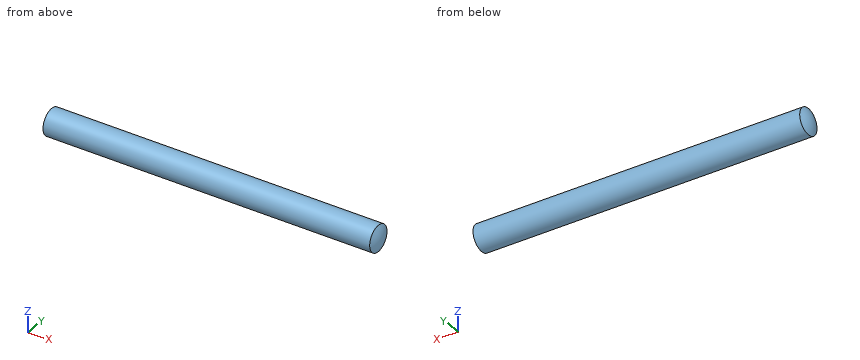
```python
from build123d import *

# Parameters (mm, degrees)
F0_R     = 4
F1_DEPTH = 50


# Not quite as in the source:
# - a pattern or mirror of a feature is missing from the dataset's text; its kind, count and spacing are read off the source's solid


with BuildPart() as f1:
    # F0 (on Right) → F1 (new body, symmetric)
    with BuildSketch(Plane.YZ):
        Circle(F0_R)
    extrude(amount=F1_DEPTH, both=True)

    # F2 (on Front) → F3 (revolve)
    with BuildSketch(Plane.XZ):
        with BuildLine():
            ThreePointArc((51.0717967697, 0), (50.79920338, 2.0705523608), (50, 4))
            Line((50, 4), (50, 0))
            Line((50, 0), (51.0717967697, 0))
        make_face()
    f3 = revolve(axis=Axis((0, 0, 0), (1, 0, 0)))

    # F3_copies: F3 across plane
    add(f3.mirror(Plane(origin=(0, 0, 0), x_dir=(0, 0, -1), z_dir=(-1, 0, 0))))


solid = f1.part
```
Geometry check sheet. Reference: the model listing, model coordinates, mm. Coordinates: 2 decimals unless noted, no trailing zeros. Write each loop counter-clockwise with the first axis right and the second up, starting at its lowest first coordinate (ties: lowest second). Pieces come first, ordered by that corner, then holes. Notation, with made-up numbers: M 14,26.25 L 49,26.25 A31 cw 49,50.25 Z; hole C 14.5,-14 d5. An arc over 180 degrees is marked long. One line per item, written item: value. Start each with the question number.
(1) Sectioned sample at A-A, the plane x = -40.5. Enter the section's corners in (y, z), and give its area (3 significant figures).
(2) Scan lines: line 1 along X through (y, z) = (0.5, 0.25); line 2 along Z through (x, y) = (-18.5, -3); line 3 along Y through (x, z) = (13.5, 1). Record each from-to range of solid material in increasing order. Write a range as [from, to].
(3) Depth check by flat-ended pin: pin 1 (3 mm diameter, centred on y = 3, z = 0.5, fed in from +X); pin 2 (2 mm diameter, centred on x = 36, y = -2, fed in from -Z); pin 3 (1.5 mm diameter, centred on y = -1, z = -1.5, fed in from -X). Enter the tip coordinate at first touch or a pass-through.
(4) Sectioned sample at B-B, the plane y = -2.25. Enter the section's corners in (x, z).
Filled sheet:
1. outline: C 0,0 d8
1. area: 50.3 mm²
2. line 1: [-51.05, 51.05]
2. line 2: [-2.65, 2.65]
2. line 3: [-3.87, 3.87]
3. pin 1: x = 50.92
3. pin 2: z = -3.87
3. pin 3: x = -51
4. outline: M -50,-3.31 L 50,-3.31 A7.68 ccw 50,3.31 L -50,3.31 A7.68 ccw Z
